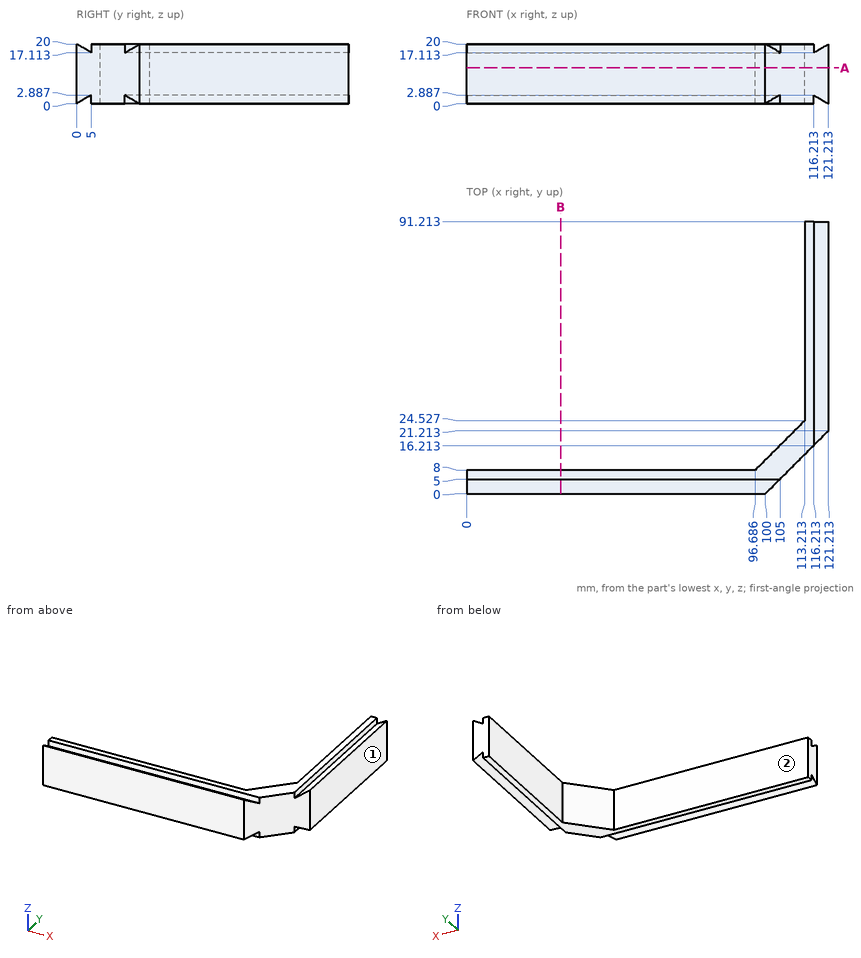
Could you check a few things on this drawing? It's one solid part, dimensions in mm from its lowest x, y, z. A direction names the side the tool comes from. Give positions to 0.01 mm unless a question says otherwise; leave off trailing zeros. Loops run counter-clockwise (first coordinate to the right, second up) from the corner with the lowest first, then second, coordinate; pieces in that order, holes last. Notation, with made-up numbers: M 54,34.5 L 73,34.5 A25 ccw 73,48.5 Z; hole C 72.25,-7 d7. An arc over 180 degrees is marked long. Return JSON: item names as keys, results as strings.
Item 1: I'm going to push flat-ended pins straight in: pin 1 Ø3 at (x, z) = (18.5, 11.5) entering from +Y; pin 2 Ø10 at (y, z) = (69, 7) entering from -X; pin 3 Ø2 at (y, z) = (11.5, 3) entering from -X. Where does each tip first touch, or does it pass through?
A:
{"pin 1": "stops at y = 8", "pin 2": "stops at x = 113.21", "pin 3": "stops at x = 99.19"}
Item 2: Please list where these lines run through material, in increasing order: line 1 (X direction, y = 48, z = 12.5); line 2 (Y direction, x = 7.5, z = 12.25); line 3 (X direction, y = 82, z = 18.25) (1 decimal).
A:
{"line 1": "x = 113.21 to 121.21", "line 2": "y = 0 to 8", "line 3": "x = 113.2 to 116.2, 118.2 to 121.2"}
Item 3: On a 3-axis mill with a long thin cutter (end or side, diameter ignored), from which of +Z, -Z, +X, -X, +Y, -Y can I reach the whole of each face in a straight line? I mean the marked faces 1 and 2. Say none if no direction works.
A:
{"face 1": "+Z, -Z, +X, +Y, -Y", "face 2": "+Z, -Z, -X, +Y"}
Item 4: Imagine slicing it at A-A on z = 12. List the corners of the cut face in (x, y) for me.
A:
{"outline": "M 0,0 L 100,0 L 121.21,21.21 L 121.21,91.21 L 113.21,91.21 L 113.21,24.53 L 96.69,8 L 0,8 Z"}
Item 5: Imagine slicing it at B-B on x = 31.5. List the corners of the cut face in (y, z) for me.
A:
{"outline": "M 0,0 L 5,2.89 L 5,0 L 8,0 L 8,20 L 5,20 L 5,17.11 L 0,20 Z"}
